from build123d import *

# Parameters (mm, degrees)
SKETCH1_R                = 30
SKETCH1_R_2              = 25
BOSS_EXTRUDE1_DEPTH      = 15.24
BOSS_EXTRUDE2_DEPTH      = 15.24
SKETCH3_R                = 10.16
BOSS_EXTRUDE3_DEPTH      = 10
BOSS_EXTRUDE3_DEPTH_BACK = 15.24
SKETCH14_R               = 38.1
SKETCH14_R_2             = 28.702
CUT_EXTRUDE1_DEPTH       = 0.89229946
CUT_EXTRUDE1_DEPTH_BACK  = 6.22629946
CUT_EXTRUDE2_DEPTH       = 6.35
SKETCH19_R               = 2.032
CUT_EXTRUDE3_DEPTH       = 18.89
SKETCH20_R               = 6.052064437
CUT_EXTRUDE4_DEPTH       = 15.24


with BuildPart() as part:
    # Sketch1 → Boss-Extrude1 (new body)
    with BuildSketch(Plane(origin=(0, 0, 0), x_dir=(1, 0, 0), z_dir=(0, 1, 0))):
        Circle(SKETCH1_R)
        Circle(SKETCH1_R_2, mode=Mode.SUBTRACT)
    extrude(amount=BOSS_EXTRUDE1_DEPTH)

    # Sketch2 → Boss-Extrude2 (add)
    with BuildSketch(Plane(origin=(0, 15.24, 0), x_dir=(1, 0, 0), z_dir=(0, 1, 0))):
        Polygon((3.584352377, -0.200805771), (0.201044225, 3.588608735), (-3.584352377, 0.200805771), (-0.201044225, -3.588608735), align=None)
        with BuildLine():
            ThreePointArc((20.22640903, 14.693276617), (18.628907162, 16.672246937), (16.838608452, 18.478670552))
            Line((16.838608452, 18.478670552), (0.201044225, 3.588608735))
            Line((0.201044225, 3.588608735), (3.584352377, -0.200805771))
            Line((3.584352377, -0.200805771), (20.22640903, 14.693276617))
        make_face()
        with BuildLine():
            Line((-3.584352377, 0.200805771), (0.201044225, 3.588608735))
            Line((0.201044225, 3.588608735), (-14.669262011, 20.243832445))
            ThreePointArc((-14.669262011, 20.243832445), (-16.650126818, 18.648680301), (-18.458673848, 16.860526676))
            Line((-18.458673848, 16.860526676), (-3.584352377, 0.200805771))
        make_face()
        with BuildLine():
            Line((-0.201044225, -3.588608735), (-3.584352377, 0.200805771))
            Line((-3.584352377, 0.200805771), (-20.22640903, -14.693276617))
            ThreePointArc((-20.22640903, -14.693276617), (-18.628907162, -16.672246937), (-16.838608452, -18.478670552))
            Line((-16.838608452, -18.478670552), (-0.201044225, -3.588608735))
        make_face()
        with BuildLine():
            Line((18.458673848, -16.860526676), (3.584352377, -0.200805771))
            Line((3.584352377, -0.200805771), (-0.201044225, -3.588608735))
            Line((-0.201044225, -3.588608735), (14.669262011, -20.243832445))
            ThreePointArc((14.669262011, -20.243832445), (16.650126818, -18.648680301), (18.458673848, -16.860526676))
        make_face()
    extrude(amount=-BOSS_EXTRUDE2_DEPTH)

    # Sketch3 → Boss-Extrude3 (add, two sides)
    with BuildSketch(Plane(origin=(0, 0, 0), x_dir=(-1, 0, 0), z_dir=(0, -1, 0))) as boss_extrude3_sk:
        Circle(SKETCH3_R)
    extrude(amount=BOSS_EXTRUDE3_DEPTH)
    extrude(boss_extrude3_sk.sketch, amount=-BOSS_EXTRUDE3_DEPTH_BACK)

    # Sketch14 → Cut-Extrude1 (cut, two sides)
    with BuildSketch(Plane(origin=(0, 10.2489, 0), x_dir=(1, 0, 0), z_dir=(0, 1, 0))) as cut_extrude1_sk:
        Circle(SKETCH14_R)
        Circle(SKETCH14_R_2, mode=Mode.SUBTRACT)
    extrude(amount=CUT_EXTRUDE1_DEPTH, mode=Mode.SUBTRACT)
    extrude(cut_extrude1_sk.sketch, amount=-CUT_EXTRUDE1_DEPTH_BACK, mode=Mode.SUBTRACT)

    # Sketch18 → Cut-Extrude2 (cut)
    with BuildSketch(Plane.XZ.offset(10)):
        Polygon((7.18570145, 0), (3.592850725, 6.223), (-3.592850725, 6.223), (-7.18570145, 0), (-3.592850725, -6.223), (3.592850725, -6.223), align=None)
    extrude(amount=-CUT_EXTRUDE2_DEPTH, mode=Mode.SUBTRACT)

    # Sketch19 → Cut-Extrude3 (cut)
    with BuildSketch(Plane.XZ.offset(3.65)):
        Circle(SKETCH19_R)
    extrude(amount=-CUT_EXTRUDE3_DEPTH, mode=Mode.SUBTRACT)

    # Sketch20 → Cut-Extrude4 (cut)
    with BuildSketch(Plane(origin=(0, 15.24, 0), x_dir=(1, 0, 0), z_dir=(0, 1, 0))):
        Circle(SKETCH20_R)
    extrude(amount=-CUT_EXTRUDE4_DEPTH, mode=Mode.SUBTRACT)


solid = part.part
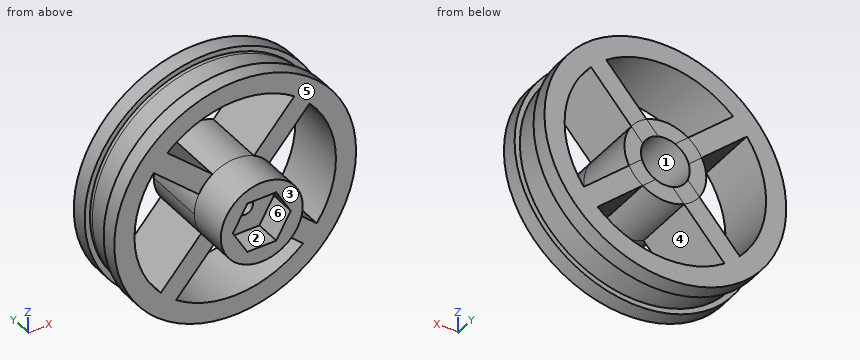
CAD build for the part. Positions are in the model's coordinates, mm. Face numbers are marked on the shaded views. A direction names the side the tool comes from. Round coordinates to 2 decimals unless told otherwise and drop trailing zeros. Order: outer loops, then holes, each group sorted by start corner. A loop starts at its lowest first (then second) coordinate and runs counter-clockwise, first axis right, second up. Notation, with made-up numbers: (3.5, 10) - (42.5, 10) arc R7 ccw to (42.5, 19) - close; hole circle Ø10 at (0.5, 8.25). An arc over 180 degrees is marked (long way). Return JSON: item names as keys, results as strings.
(1) Cut at B-B (x = 0). State how many separate pieces and enclosed holes the cut face has, then the cut area to 3 significant figures.
Answer key:
{"separate pieces": "4", "enclosed holes": "0", "area": "368 mm^2"}
(2) Cut at D-D (z = -13). Give the cut face in (x, y), then the cut area to 3 significant figures.
Answer key:
{"outline": "(-27.04, 0) - (-21.35, 0) - (-21.35, 15.24) - (-27.04, 15.24) - (-27.04, 11.14) - (-25.59, 11.14) - (-25.59, 4.02) - (-27.04, 4.02) - close; (-15.01, 0) - (-8.2, 0) - (-8.2, 15.24) - (-15.01, 15.24) - close; (10.72, 0) - (18.33, 0) - (18.33, 15.24) - (10.72, 15.24) - close; (21.35, 0) - (27.04, 0) - (27.04, 4.02) - (25.59, 4.02) - (25.59, 11.14) - (27.04, 11.14) - (27.04, 15.24) - (21.35, 15.24) - close", "area": "372 mm^2"}
(3) Cut at C-C (y = -8). Give the cut face in (x, z).
Answer key:
{"outline": "circle Ø20.32 at (0, 0); hole (-7.19, 0) - (-3.59, -6.22) - (3.59, -6.22) - (7.19, 0) - (3.59, 6.22) - (-3.59, 6.22) - close"}
(4) Pin check, flat tips, straight feed: pin 1 Ø9.5 at (x, z) = (0, 0) entering from -Y; pin 2 Ø1 at (y, z) = (6, -1) entering from +X; pin 3 Ø5 at (x, y) = (15.5, 4.5) entering from +Z; pin 4 Ø5 at (x, z) = (-16, 4.5) entering from -Y. Stop position of each tip, or through.
Answer key:
{"pin 1": "stops at y = -3.65", "pin 2": "stops at x = 28.7", "pin 3": "stops at z = 27.01", "pin 4": "passes through"}
(5) Wall check: probe 1 along Z at (x, y) = (0, 5); probe 2 along Z at (x, y) = (-10.5, 1). Give the ranges that are in metal, low to high. Write a range as from..to.
Answer key:
{"probe 1": "z = -28.7..-25, -10.16..-6.05, 6.05..10.16, 25..28.7", "probe 2": "z = -28.1..-22.69, -15.57..-7.95, 5.99..12.81, 22.69..28.1"}
(6) Cut at A-A (y = 2.75). Give the cut face in (x, z).
Answer key:
{"outline": "circle Ø60 at (0, 0); hole (-20.23, 14.69) arc R25 ccw to (-18.46, -16.86) - (-8.45, -5.65) arc R10.16 cw to (-9.02, 4.67) - close; hole (-16.84, 18.48) - (-5.64, 8.45) arc R10.16 cw to (4.66, 9.03) - (14.67, 20.24) arc R25 ccw to start; hole (-14.67, -20.24) arc R25 ccw to (16.84, -18.48) - (5.64, -8.45) arc R10.16 cw to (-4.66, -9.03) - close; hole circle Ø12.1 at (0, 0); hole (8.45, 5.65) arc R10.16 cw to (9.02, -4.67) - (20.23, -14.69) arc R25 ccw to (18.46, 16.86) - close"}
(7) Tool access for the marked faces 1, 2, 3 and 4: list every direction of +Z, -Z, +X, -X, +Y, -Y with a clear straight run to the whole face (end or side of a thin tool).
Answer key:
{"face 1": "+Y", "face 2": "-Y", "face 3": "+Z, -Z, +X, -X, -Y", "face 4": "+Y, -Y"}
(8) Pull direction X, two halves, no side cores. Call the marked faces 5 and 6: +X half, -X half, draft (parallel to the pull), parting line (faces both ways), or undercut.
Answer key:
{"face 5": "draft", "face 6": "undercut"}
